The drawing under review shows one solid part. Ordinate dimensions are in mm from its lowest x, y, z. A direction names the side the tool comes from. Coordinates: 2 decimals unless noted, no trailing zeros. Order: outer loops, then holes, each group sorted by start corner. A loop starts at its lowest first (then second) coordinate and runs counter-clockwise, first axis right, second up.
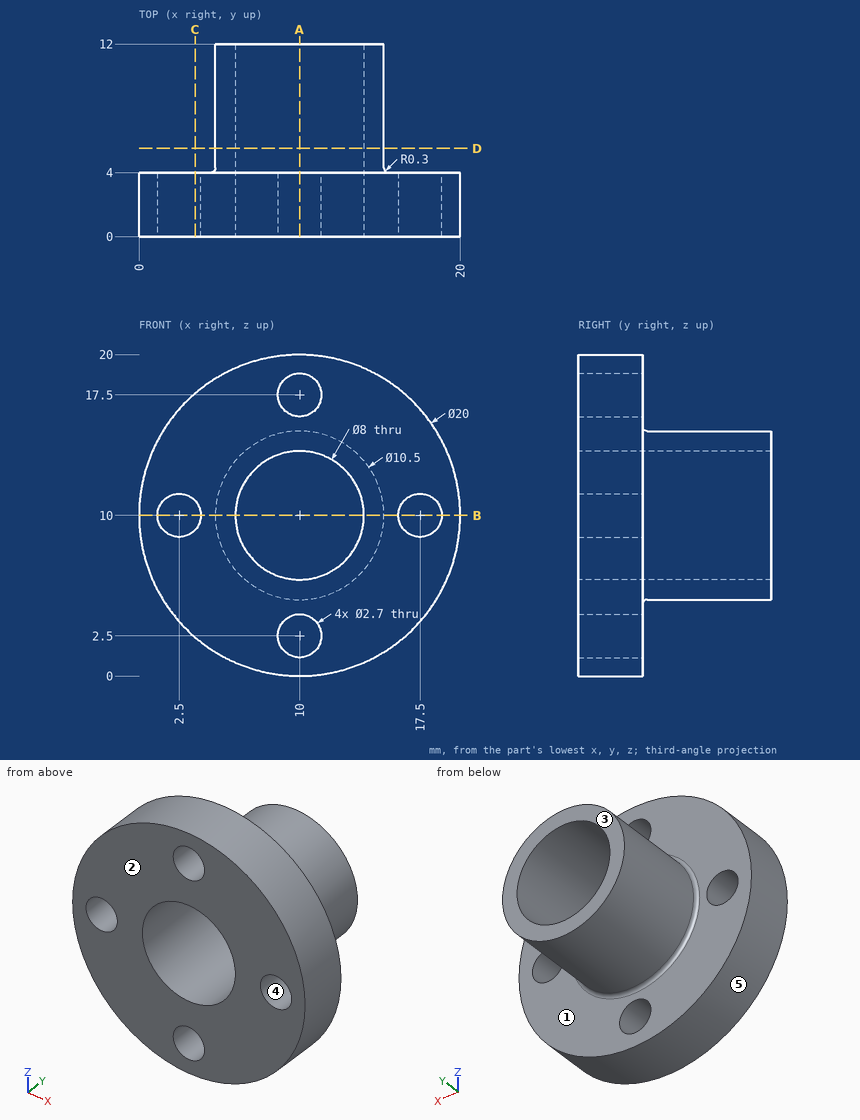
(1) We need section C-C, the plane x = 3.5. Write out the cut boundary in (y, z).
A:
outline: (0, 2.4) - (4, 2.4) - (4, 9.09) - (0, 9.09) - close; (0, 10.91) - (4, 10.91) - (4, 17.6) - (0, 17.6) - close
(2) Machinability: for the marked faces 1 and 2, which of the approach directions +Z, -Z, +X, -X, +Y, -Y give a long, thin tool a straight path to every point of the face, cutting with its end or side? Answer none if there is none.
A:
face 1: +Y
face 2: +Z, -Z, +X, -X, -Y
(3) We need section B-B, the plane z = 10. Write out the cut boundary in (x, y), and give its area (3 significant figures).
A:
outline: (0, 0) - (1.15, 0) - (1.15, 4) - (0, 4) - close; (3.85, 0) - (6, 0) - (6, 12) - (4.75, 12) - (4.75, 4.3) arc R0.3 cw to (4.45, 4) - (3.85, 4) - close; (14, 0) - (16.15, 0) - (16.15, 4) - (15.55, 4) arc R0.3 cw to (15.25, 4.3) - (15.25, 12) - (14, 12) - close; (18.85, 0) - (20, 0) - (20, 4) - (18.85, 4) - close
area: 46.4 mm2
(4) Draft analysis for pull direction Z (two halves, no side actions). For the marked faces 3, 4 and 5, state which applies: released by +Z, released by -Z, zero draft, split by the parting line, or undercut.
A:
face 3: zero draft
face 4: undercut
face 5: split by the parting line
(5) We need section D-D, the plane y = 5.5. Write out the cut boundary in (x, z).
A:
outline: circle Ø10.5 at (10, 10); hole circle Ø8 at (10, 10)
(6) Wall thickness on probe 1 along Z at (x, y) = (10, 4.25); probe 2 along Y at (x, z) = (4.5, 16.75): over which ranges is each line inside the solid? List them lowest first.
A:
probe 1: z = 4.75 to 6, 14 to 15.25
probe 2: y = 0 to 4
(7) For pin 1 Ø8 at (x, z) = (4.5, 6.5) entering from +Y; pin 2 Ø2 at (x, z) = (2.5, 10) entering from -Y; pin 3 Ø1 at (x, z) = (5, 3.5) entering from +Y; pin 4 Ø4 at (y, z) = (7, 5.5) entering from +X, all flat-tipped, find the tip position at first contact; note any pin that passes through.
A:
pin 1: stops at y = 12
pin 2: passes through
pin 3: stops at y = 4
pin 4: stops at x = 14.62
(8) We need section A-A, the plane x = 10. Write out the cut boundary in (y, z), and give its area (3 significant figures).
A:
outline: (0, 0) - (4, 0) - (4, 1.15) - (0, 1.15) - close; (0, 3.85) - (4, 3.85) - (4, 4.45) arc R0.3 cw to (4.3, 4.75) - (12, 4.75) - (12, 6) - (0, 6) - close; (0, 14) - (12, 14) - (12, 15.25) - (4.3, 15.25) arc R0.3 cw to (4, 15.55) - (4, 16.15) - (0, 16.15) - close; (0, 18.85) - (4, 18.85) - (4, 20) - (0, 20) - close
area: 46.4 mm2
